from build123d import *

# Parameters (mm, degrees)
BOSS_EXTRUDE2_DEPTH = 25
BOSS_EXTRUDE4_DEPTH = 5
BOSS_EXTRUDE5_DEPTH = 15


with BuildPart() as part:
    # Sketch1 → Boss-Extrude2 (new body)
    with BuildSketch(Plane(origin=(0, 0, 0), x_dir=(1, 0, 0), z_dir=(0, 1, 0))):
        Polygon((0, 0), (15, 0), (15, 6.5), (11, 6.5), (11, 5), (13, 5), (13, 2), (2, 2), (2, 5), (4, 5), (4, 6.5), (0, 6.5), align=None)
    extrude(amount=BOSS_EXTRUDE2_DEPTH)

    # Sketch3 → Boss-Extrude4 (add)
    with BuildSketch(Plane.XY):
        with BuildLine():
            Line((15, 25), (15, 28.291553618))
            Line((15, 28.291553618), (15, 30.5))
            ThreePointArc((15, 30.5), (14.62928544, 32.855859369), (13.53772985, 34.976238828))
            Line((13.53772985, 34.976238828), (10.707203961, 32.890364565))
            ThreePointArc((10.707203961, 32.890364565), (7.504387795, 26.542932427), (4.28759779, 32.883294263))
            Line((4.28759779, 32.883294263), (1.455694475, 34.967301819))
            ThreePointArc((1.455694475, 34.967301819), (0.3689938, 32.850585244), (0, 30.5))
            Line((0, 30.5), (0, 28.291553618))
            Line((0, 28.291553618), (0, 25))
            Line((0, 25), (0, 15))
            Line((0, 15), (15, 15))
            Line((15, 15), (15, 25))
        make_face()
    extrude(amount=BOSS_EXTRUDE4_DEPTH)

    # Sketch4 → Boss-Extrude5 (add)
    with BuildSketch(Plane(origin=(15, 0, 0), x_dir=(0, 0, -1), z_dir=(1, 0, 0))):
        Polygon((-5, 15), (0, 10), (0, 15), align=None)
    extrude(amount=-BOSS_EXTRUDE5_DEPTH)


solid = part.part
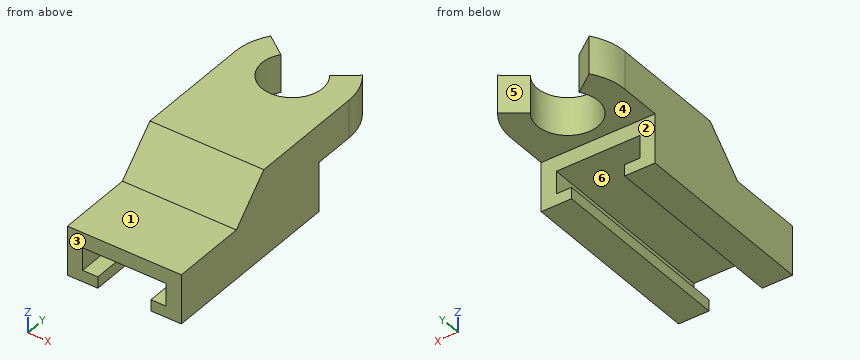
Geometry check sheet. Reference: the model listing, model coordinates, mm. Face numbers are marked on the shaded views. A direction names the side the tool comes from. Give positions to 0.01 mm unless a question says otherwise; leave off trailing zeros. Write each loop counter-clockwise with the first axis right and the second up, starting at its lowest first coordinate (ties: lowest second). Pieces come first, ordered by that corner, then holes. Notation, with made-up numbers: (-24.75, 22) - (0.25, 22) arc R34 ccw to (0.25, 56) - close; hole circle Ø6 at (58, 30). An arc over 180 degrees is marked (long way). Put each result on its own line as item: value.
1. Sectioned sample at C-C, the plane z = 4. Enter the section's corners in (x, y), plus the area to 3 significant figures.
Ans:
outline: (0, 14) - (15, 14) - (15, 30.5) arc R7.5 ccw to (13.54, 34.98) - (10.71, 32.89) arc R3.98 cw (long way) to (4.29, 32.88) - (1.46, 34.97) arc R7.5 ccw to (0, 30.5) - close
area: 249 mm²
2. Draft check along Z on the marked faces 4, 5 and 6. Enter one of: +Z half, -Z half, draft (parallel to the pull), parting line (faces both ways), or undercut.
Ans:
face 4: -Z half
face 5: draft
face 6: undercut
3. Sectioned sample at D-D, the plane x = 12. Enter the section's corners in (y, z).
Ans:
outline: (0, -6.5) - (25, -6.5) - (25, -5) - (0, -5) - close; (0, -2) - (25, -2) - (25, 0) - (33.84, 0) - (33.84, 5) - (15, 5) - (10, 0) - (0, 0) - close
4. Sectioned sample at A-A, the plane y = 13. Enter the section's corners in (x, z), plus the area to 3 significant figures.
Ans:
outline: (0, -6.5) - (4, -6.5) - (4, -5) - (2, -5) - (2, -2) - (13, -2) - (13, -5) - (11, -5) - (11, -6.5) - (15, -6.5) - (15, 3) - (0, 3) - close
area: 99.0 mm²
5. Thickness scan on line 1 (X direction, y = 11.5, z = -4.25); line 2 (Z direction, x = 5.5, y = 27); line 3 (Z direction, x = 2.25, y = 19). Record the ranges inside material, lowest first.
Ans:
line 1: x = 0 to 2, 13 to 15
line 2: z = 0 to 5
line 3: z = -6.5 to -5, -2 to 5
6. Sectioned sample at B-B, the plane x = 7.5. Enter the section's corners in (y, z).
Ans:
outline: (0, -2) - (25, -2) - (25, 0) - (26.54, 0) - (26.54, 5) - (15, 5) - (10, 0) - (0, 0) - close
7. Go/stop test with flat-tipped pins: pin 1 (1.6 mm diameter, centred on x = 12.5, y = 10.5, fed in from +Z); pin 2 (8 mm diameter, centred on x = 6.5, y = 31.5, fed in from -Z); pin 3 (2 mm diameter, centred on x = 13.5, y = 13.5, fed in from +Z). Record where each tip stops, or that it passes through.
Ans:
pin 1: stops at z = 1.3
pin 2: stops at z = 0
pin 3: stops at z = 4.5
8. Set-up check for the marked faces 1, 2 and 3: record each of +Z, -Z, +X, -X, +Y, -Y from which the full face is reachable in a straight line by a thin tool's end or side.
Ans:
face 1: +Z, +X, -X, -Y
face 2: -Z, +X, -X, +Y
face 3: +Z, -Z, +X, -X, -Y
